Autodesk Inventor part; units mm, degrees
ref_plane "YZ Plane" through (0, 0, 0) normal (1, 0, 0) x (0, 1, 0)
ref_plane "XZ Plane" through (0, 0, 0) normal (0, 1, 0) x (-1, 0, 0)
ref_plane "XY Plane" through (0, 0, 0) normal (0, 0, 1) x (1, 0, 0)
ref_plane "작업 평면1" through (0, 0, 0) normal (0, 0, 1) x (1, 0, 0)
ref_plane "작업 평면2" through (-17, 0, 48.4) normal (-1, 0, 0) x (0, 0, 1)
sketch "스케치2" plane through (-17, 0, 48.4) normal (-1, 0, 0) x (0, 0, 1)
  line L0 (13.5, -39.75) -> (11.5, -39.75)
  arc A0 (11.5, -39.75) -> (9.25, -42) centre (11.5, -42) ccw
  line L1 (9.25, -42) -> (9.25, -44)
  arc A1 (8.25, -45) -> (9.25, -44) centre (8.25, -44) ccw
  line L2 (8.25, -45) -> (-8.25, -45)
  arc A2 (-9.25, -44) -> (-8.25, -45) centre (-8.25, -44) ccw
  line L3 (-9.25, -44) -> (-9.25, -42)
  arc A3 (-9.25, -42) -> (-11.5, -39.75) centre (-11.5, -42) ccw
  line L4 (-11.5, -39.75) -> (-13.5, -39.75)
  arc A4 (-14.5, -38.75) -> (-13.5, -39.75) centre (-13.5, -38.75) ccw
  line L5 (-14.5, -38.75) -> (-14.5, 8.25)
  arc A5 (-13.5, 9.25) -> (-14.5, 8.25) centre (-13.5, 8.25) ccw
  line L6 (-13.5, 9.25) -> (-11.5, 9.25)
  arc A6 (-11.5, 9.25) -> (-9.25, 11.5) centre (-11.5, 11.5) ccw
  line L7 (-9.25, 11.5) -> (-9.25, 14.5)
  line L8 (-15, 14.5) -> (-9.25, 14.5)
  line L9 (-20.1, 8.5) -> (-15, 14.5)
  line L10 (-20.1, -44.6) -> (-20.1, 8.5)
  line L11 (-15, -50.6) -> (-20.1, -44.6)
  line L12 (15, -50.6) -> (-15, -50.6)
  line L13 (20.1, -44.6) -> (15, -50.6)
  line L14 (20.1, 8.5) -> (20.1, -44.6)
  line L15 (15, 14.5) -> (20.1, 8.5)
  line L16 (9.25, 14.5) -> (15, 14.5)
  line L17 (9.25, 14.5) -> (9.25, 11.5)
  arc A7 (9.25, 11.5) -> (11.5, 9.25) centre (11.5, 11.5) ccw
  line L18 (11.5, 9.25) -> (13.5, 9.25)
  arc A8 (14.5, 8.25) -> (13.5, 9.25) centre (13.5, 8.25) ccw
  line L19 (14.5, 8.25) -> (14.5, -38.75)
  arc A9 (13.5, -39.75) -> (14.5, -38.75) centre (13.5, -38.75) ccw
  circle A10 centre (17.3, 4) radius 1.35
  circle A11 centre (17.3, -18) radius 1.35
  circle A12 centre (11, -47.8) radius 1.35
  circle A13 centre (-17.3, 4) radius 1.35
  circle A14 centre (-17.3, -18) radius 1.35
  circle A15 centre (-11, -47.8) radius 1.35
  circle A16 centre (17.3, -40) radius 1.35
  circle A17 centre (-17.3, -40) radius 1.35
  circle A18 centre (-17.3, -18) radius 2.8
  circle A19 centre (-17.3, 4) radius 2.8
  line L20 (-17.3, -18) -> (-17.3, 4)
  line L21 (-17.3, 4) -> (-17.3, -7)
  line L22 (-19.7531, 5.35) -> (-19.7531, -19.35)
  line L23 (-19.7531, -19.35) -> (-14.8469, -19.35)
  line L24 (-14.8469, -19.35) -> (-14.8469, 5.35)
  line L25 (-14.8469, 5.35) -> (-19.7531, 5.35)
  line L26 (-19.7531, 5.35) -> (-14.8469, -19.35) construction
  line L27 (-19.7531, -19.35) -> (-14.8469, 5.35) construction
  point P0 (-48.4, 0)
  point P1 (-19.7531, -19.35)
  point P2 (-14.8469, -19.35)
  point P3 (-14.8469, 5.35)
  point P4 (-19.7531, 5.35)
  dimension "d0" = 11
extrude "돌출1" add sketch "스케치2" along normal blind 3.1 contours A18 L23 | L23 A14 L20 A18 L24 | A18 L20 A19 L24 | L25 A19 | L24 A19 L20 A13 L25 | L22 A18 L20 A14 L23 | A18 L22 A19 L20 | L25 A13 L20 A19 L22
sketch "스케치3" plane through (-17, -19.35, 28.6469) normal (0, 0, -1) x (-1, 0, 0)
  line L0 (3.1, 24.7) -> (3.1, 0)
  line L1 (0, 0) -> (3.1, 0)
  line L2 (0, 24.7) -> (0, 0)
  line L3 (0, 0) -> (3.1, 0)
  line L4 (3.1, 24.7) -> (3.1, 0)
  line L5 (0, 24.7) -> (3.1, 24.7)
  point P0 (-17, 19.35)
extrude "돌출2" add sketch "스케치3" along normal blind 0.347
sketch "스케치4" plane through (-17, -19.35, 28.2999) normal (0, 0, -1) x (-1, 0, 0)
  line L0 (-4.5, 27.325) -> (-4.5, 25.825)
  line L1 (-4.5, 25.825) -> (-2.5, 25.825)
  line L2 (-2.5, 20.875) -> (-2.5, 25.825)
  line L3 (-4.5, 20.875) -> (-2.5, 20.875)
  line L4 (-4.5, 20.875) -> (-4.5, 19.375)
  line L5 (-4.5, 19.375) -> (-2, 19.375)
  line L6 (-2, 5.325) -> (-2, 19.375)
  line L7 (-2, 5.325) -> (-4.5, 5.325)
  line L8 (-4.5, 5.325) -> (-4.5, 3.825)
  line L9 (-4.5, 3.825) -> (-2.5, 3.825)
  line L10 (-2.5, -1.125) -> (-2.5, 3.825)
  line L11 (-4.5, -1.125) -> (-2.5, -1.125)
  line L12 (-4.5, -1.125) -> (-4.5, -2.625)
  line L13 (-4.5, -2.625) -> (-2, -2.625)
  line L14 (-2, -16.675) -> (-2, -2.625)
  line L15 (-2, -16.675) -> (-4.5, -16.675)
  line L16 (-4.5, -16.675) -> (-4.5, -18.175)
  line L17 (-4.5, -18.175) -> (-2.5, -18.175)
  line L18 (-2.5, -23.125) -> (-2.5, -18.175)
  line L19 (-4.5, -23.125) -> (-2.5, -23.125)
  line L20 (-4.5, -23.125) -> (-4.5, -24.625)
  line L21 (-4.5, -24.625) -> (-2, -24.625)
  line L22 (-2, -25.25) -> (-2, -24.625)
  line L23 (-2, -25.25) -> (0, -25.25)
  line L24 (0, -25.25) -> (0, 27.85)
  line L25 (-2, 27.85) -> (0, 27.85)
  line L26 (-2, 27.325) -> (-2, 27.85)
  line L27 (-2, 27.325) -> (-4.5, 27.325)
  line L28 (0, 0) -> (3.1, 0)
  line L29 (-2.5, 0) -> (0, 0)
  line L30 (3.1, 24.7) -> (0, 24.7)
  line L31 (-2.5, 24.7) -> (0, 24.7)
  line L32 (3.1, -2.625) -> (-2.5, -2.625)
  line L33 (-2.5, 27.325) -> (1.417, 27.325)
  line L34 (3.1, 24.7) -> (-2.5, 24.7)
  line L35 (-2.5, 24.7) -> (-2.5, 27.325)
  line L36 (-2.5, 27.325) -> (3.1, 27.325)
  line L37 (3.1, 27.325) -> (3.1, 24.7)
  line L38 (-2.5, 0) -> (3.1, 0)
  line L39 (3.1, 0) -> (3.1, -2.625)
  line L40 (3.1, -2.625) -> (-2.5, -2.625)
  line L41 (-2.5, -2.625) -> (-2.5, 0)
  line L42 (3.1, 23.9266) -> (3.1, -20.3266)
  line L43 (3.1, 0) -> (3.1, 24.7)
  circle A0 centre (0.3, 1.35) radius 1.35
  circle A1 centre (0.3, 23.35) radius 1.35
  point P0 (-17, 19.35)
  point P1 (1.417, 27.325)
  point P2 (-2.5, 25.825)
  point P3 (-2.5, -1.125)
  point P4 (-2.5, -2.625)
  point P5 (0.3, 24.7)
  point P6 (0, 24.6662)
  point P7 (0, 0.0338)
  point P8 (0.3, 0)
extrude "돌출3" add sketch "스케치4" along normal blind 28.3 contours L27 L33 L24 L31 L2 L35 | L31 L24 A1 A0 L29 L10 L9 L8 L7 L6 L5 L4 L3 L2 | L33 L36 L37 L30 L24 | L30 L43 L42 L28 A0 L24 A1 | L39 L32 L24 L28 | L24 L32 L13 L41 L10 L29
sketch "스케치6" plane through (-17, -19.35, -0.0001) normal (0, 0, -1) x (-1, 0, 0)
  point P0 (-17, 19.35)
sketch "스케치7" plane through (-20.1, 0, 48.4) normal (-1, 0, 0) x (0, 0, 1)
  line L0 (-20.1001, -15.525) -> (-48.4001, -15.525)
  line L1 (-20.1001, -19.35) -> (-48.4001, -19.35)
  line L2 (-48.4001, 2.65) -> (-20.1001, 2.65)
  line L3 (-20.1001, 5.35) -> (-48.4001, 5.35)
  line L4 (-48.4001, -19.35) -> (-45.4001, -19.35)
  line L5 (-45.4001, -19.35) -> (-45.4001, 5.35)
  line L6 (-43.3972, -19.35) -> (-43.3972, -17.4375)
  line L7 (-43.3972, -17.4375) -> (-45.4001, -17.4375)
  line L8 (-46.4001, -14.9375) -> (-46.4001, -19.9375)
  line L9 (-46.4001, -19.9375) -> (-44.4001, -19.9375)
  line L10 (-44.4001, -19.9375) -> (-44.4001, -14.9375)
  line L11 (-44.4001, -14.9375) -> (-46.4001, -14.9375)
  line L12 (-46.4001, -14.9375) -> (-44.4001, -19.9375) construction
  line L13 (-46.4001, -19.9375) -> (-44.4001, -14.9375) construction
  line L14 (-45.4001, 2.65) -> (-45.4001, 4)
  line L15 (-46.4001, 6.5) -> (-46.4001, 1.5)
  line L16 (-46.4001, 1.5) -> (-44.4001, 1.5)
  line L17 (-44.4001, 1.5) -> (-44.4001, 6.5)
  line L18 (-44.4001, 6.5) -> (-46.4001, 6.5)
  line L19 (-46.4001, 6.5) -> (-44.4001, 1.5) construction
  line L20 (-46.4001, 1.5) -> (-44.4001, 6.5) construction
  point P0 (-48.4, 0)
  dimension "d7" = 3
  dimension "d8" = 1.9125
  dimension "d9" = 2
  dimension "d10" = 1.35
  dimension "d11" = 5
  dimension "d12" = 5
  dimension "d13" = 2
extrude "돌출4" cut sketch "스케치7" against normal blind 6 contours L10 L7 L5 L0 | L16 L15 L2 L5 | L5 L2 L17 L16 | L0 L5 L11 L10 | L5 L1 L8 L0 | L0 L8 L11 L5 | L10 L1 L5 L7 | L10 L9 L8 L1 | L5 L3 L17 L2 | L2 L15 L3 L5 | L15 L18 L17 L3
sketch "스케치8" plane through (-17, 0, 48.4) normal (-1, 0, 0) x (0, 0, 1)
  line L0 (-20.1001, -21.975) -> (-20.1001, -19.35)
  line L1 (-20.1001, -21.975) -> (-20.1001, 7.975)
  line L2 (-20.1001, 7.975) -> (-14.8422, 7.975)
  line L3 (-14.8422, 7.975) -> (-14.8422, -21.975)
  line L4 (-14.8422, -21.975) -> (-20.1001, -21.975)
  arc A0 (-19.7531, -19.35) -> (-14.8469, -19.35) centre (-17.3, -18) ccw
  line L5 (-19.7531, -19.35) -> (-20.1001, -19.35)
  line L6 (-20.1001, -19.3162) -> (-20.1001, -19.35)
  line L7 (-20.1001, -16.6838) -> (-20.1001, -19.3162)
  line L8 (-20.1001, 2.6838) -> (-20.1001, -16.6838)
  line L9 (-20.1001, 5.3162) -> (-20.1001, 2.6838)
  line L10 (-20.1001, 5.35) -> (-20.1001, 5.3162)
  line L11 (-19.7531, 5.35) -> (-20.1001, 5.35)
  arc A1 (-14.8469, 5.35) -> (-19.7531, 5.35) centre (-17.3, 4) ccw
  line L12 (-14.8469, -19.35) -> (-14.8469, 5.35)
  circle A2 centre (-17.3, 4) radius 1.35
  circle A3 centre (-17.3, -18) radius 1.35
  point P0 (-48.4, 0)
  point P1 (-20.1001, 5.35)
  point P2 (-20.1001, -19.35)
extrude "돌출5" add sketch "스케치8" along normal blind 3.1 contours L0 L5 A0 L12 A1 L11 L1 L2 L3 L4
sketch "스케치9" plane through (-12.5, 0.025, 28.2999) normal (1, 0, 0) x (0, 0, -1)
  line L0 (0, 1.5) -> (0, 0)
  line L1 (0, 0) -> (28.3, 0)
  line L2 (28.3, 1.5) -> (28.3, 0)
  line L3 (0, 1.5) -> (28.3, 1.5)
  line L4 (0, -14.05) -> (0, -15.55)
  line L5 (0, -15.55) -> (28.3, -15.55)
  line L6 (28.3, -14.05) -> (28.3, -15.55)
  line L7 (0, -14.05) -> (28.3, -14.05)
  point P0 (28.2999, -0.025)
extrude "돌출6" cut sketch "스케치9" against normal up to surface (2 mm away)
sketch "스케치10" plane through (-15, -14.025, 28.2999) normal (1, 0, 0) x (0, 0, -1)
  line L0 (0, 14.05) -> (0, 0)
  line L1 (0, 0) -> (28.3, 0)
  line L2 (28.3, 14.05) -> (28.3, 0)
  line L3 (0, 14.05) -> (28.3, 14.05)
  point P0 (28.2999, 14.025)
extrude "돌출7" add sketch "스케치10" along normal up to surface (0.5 mm away)
properties part number "_108-64_adt"
Geometry check sheet. Reference: the model listing, model coordinates, mm. A direction names the side the tool comes from. Coordinates: 2 decimals unless noted, no trailing zeros. Loops run counter-clockwise (first coordinate to the right, second up) from the corner with the lowest first, then second, coordinate; pieces in that order, holes last. Notation, with made-up numbers: (-35.75, 82) - (-7.75, 82) arc R37 cw to (-7.75, 121) - close; hole circle Ø11 at (46, 33.25). An arc over 180 degrees is marked (long way). Use one line per item in the form item = value. Start each with the question number.
Item 1: Section check C-C, the plane z = 16. Enter the section's corners in (x, y) (3 decimals), and give its area (3 significant figures).
Item 2: Tool access check on faces 5 (the face through (-17.508, 2.666, 16.32)), 6 (the face through (-17, -14.938, 3)), 7 (the face through (-16, -7, 28.3)). Record the directions out of +Z, -Z, +X, -X, +Y, -Y that give a thin tool (end or side, any length) a straight path to the whole face; none if there is none.
Item 3: Mould release check, pull along Z, two halves, no side actions. Record for faces 1 (the face through (-18.53, -17.18, 30.03)), 2 (the face through (-17, -16, 4)), 3 (the face through (-20.1, -7, 17)), 4 (the face through (-19, -7, 33.558)): +Z half, -Z half, draft (parallel to the pull), parting line (faces both ways), or undercut.
Item 4: Thickness scan on probe 1 along Y at (x, z) = (-19.4, 31.1) (3 decimals); probe 2 along Z at (x, y) = (-17.7, 4). Record the ranges inside material, lowest first.
Item 5: Section check B-B, the plane y = -15.5. Enter the section's corners in (x, z), and give its area (3 significant figures).
Item 6: Section check A-A, the plane z = 31.1. Enter the section's corners in (x, y) (3 decimals).
Item 7: Gauge pin test, flat ends, axial feed: pin 1 (1.5 mm diameter, centred on x = -16.5, z = 29, fed in from -Y) (3 decimals); pin 2 (0.8 mm diameter, centred on x = -18, y = 3.5, fed in from -Z). Record the tip position at first contact, or that the pin passes through.
Item 8: Section check D-D, the plane x = -16.45. Enter the section's corners in (y, z) (1 decimal).
Computed:
q1.outline = (-20.1, -21.975) - (-14.5, -21.975) - (-14.5, 7.975) - (-20.1, 7.975) - close; hole (-17.3, -19.35) - (-17, -19.35) - (-17, -19.316) arc R1.35 ccw (long way) to start; hole (-17.3, 5.35) arc R1.35 ccw (long way) to (-17, 5.316) - (-17, 5.35) - close
q1.area = 156 mm2
q2.face_5 = -Z
q2.face_6 = +X, -X
q2.face_7 = +Z, +X, +Y, -Y
q3.face_1 = undercut
q3.face_2 = undercut
q3.face_3 = draft
q3.face_4 = +Z half
q4.probe_1 = -21.975 to -19.35, -16.65 to 2.65, 5.35 to 7.975
q4.probe_2 = 28.3 to 29.75, 32.45 to 33.56
q5.outline = (-20.1, 0) - (-14.5, 0) - (-14.5, 2) - (-20.1, 2) - close; (-20.1, 4) - (-14.5, 4) - (-14.5, 28.3) - (-17, 28.3) - (-17, 33.56) - (-20.1, 33.56) - close
q5.area = 164 mm2
q6.outline = (-20.1, -21.975) - (-17, -21.975) - (-17, -19.35) - (-20.1, -19.35) - close; (-20.1, -16.65) - (-17, -16.65) - (-17, 2.65) - (-20.1, 2.65) - close; (-20.1, 5.35) - (-17, 5.35) - (-17, 7.975) - (-20.1, 7.975) - close
q7.pin_1 = -21.975
q7.pin_2 = 28.3
q8.outline = (-22, 0) - (-19, 0) - (-19, 2) - (-19.9, 2) - (-19.9, 4) - (-19, 4) - (-19, 28.3) - (-22, 28.3) - close; (-17, 0) - (3, 0) - (3, 2) - (1.5, 2) - (1.5, 4) - (3, 4) - (3, 28.3) - (-17, 28.3) - (-17, 4) - (-14.9, 4) - (-14.9, 2) - (-17, 2) - close; (5, 0) - (8, 0) - (8, 28.3) - (5, 28.3) - (5, 4) - (6.5, 4) - (6.5, 2) - (5, 2) - close
